```python
from build123d import *

# Parameters (mm, degrees)
F0_R     = 101.6
F1_DEPTH = 25.4


with BuildPart() as f1:
    # F0 (on Front) → F1 (new body)
    with BuildSketch(Plane.XZ):
        Circle(F0_R)
        Polygon((-12.69949, -19.163814), (-12.69949, -0.113814), (-12.69949, 18.936186), (12.70051, 18.936186), (12.7, -19.163814), align=None, mode=Mode.SUBTRACT)
    extrude(amount=F1_DEPTH)


solid = f1.part
```
Check sheet for the modelled part. Datum: model origin and axes. Units: mm. A direction names the side the tool comes from. Coordinates: 2 decimals unless noted, no trailing zeros. Write each loop counter-clockwise with the first axis right and the second up, starting at its lowest first coordinate (ties: lowest second). Pieces come first, ordered by that corner, then holes. Notation, with made-up numbers: (-37.5, -5.5) - (-9.5, -5.5) arc R16 ccw to (-9.5, 12.5) - close; hole circle Ø4 at (7.5, 12.25). An arc over 180 degrees is marked (long way). One line per question, with ' | ' between items.
Item 1: Access from +Z, -Z, +X, -X, +Y, -Y to the whole of each face (thin tool, end or side, straight path). Record for faces 1 (the face through (0, -13, -19.164)), 2 (the face through (21, 0, 1)).
Determined:
face 1: +Y, -Y | face 2: +Z, -Z, +X, -X, +Y
Item 2: Sectioned sample at D-D on z = -77. Record the boundary of the cut face in (x, y), plus the area to 3 significant figures.
Determined:
outline: (-66.28, -25.4) - (66.28, -25.4) - (66.28, 0) - (-66.28, 0) - close | area: 3,370 mm2
Item 3: Gauge pin test, flat ends, axial feed: P1, Ø6, axis at x = -4, z = -16, coming from the +Y side; P2, Ø6, axis at x = -25, z = 21.5, coming from the +Y side; P3, Ø5, axis at y = -10, z = 38.5, coming from the -X side; P4, Ø1.5, axis at x = 36.5, y = -3, coming from the -Z side. Record the tip position at first contact, or that the pin passes through.
Determined:
P1: passes through | P2: stops at y = 0 | P3: stops at x = -95.01 | P4: stops at z = -95.1
Item 4: Sectioned sample at A-A on x = 0. Record the boundary of the cut face in (y, z), plus the area to 3 significant figures.
Determined:
outline: (-25.4, -101.6) - (0, -101.6) - (0, -19.16) - (-25.4, -19.16) - close; (-25.4, 18.94) - (0, 18.94) - (0, 101.6) - (-25.4, 101.6) - close | area: 4,190 mm2
Item 5: Sectioned sample at B-B on z = 0. Record the boundary of the cut face in (x, y), plus the area to 3 significant figures.
Determined:
outline: (-101.6, -25.4) - (-12.7, -25.4) - (-12.7, 0) - (-101.6, 0) - close; (12.7, -25.4) - (101.6, -25.4) - (101.6, 0) - (12.7, 0) - close | area: 4,520 mm2
Item 6: Thickness scan on line 1 (Z direction, x = -18, y = -11.75); line 2 (Z direction, x = -38, y = -11.25); line 3 (X direction, y = -23.25, z = -33). Record the ranges inside material, lowest first. Write a range as [from, to].
Determined:
line 1: z = [-99.99, 99.99] | line 2: z = [-94.23, 94.23] | line 3: x = [-96.09, 96.09]
Item 7: Mould release check, pull along Z, two halves, no side actions. Record for faces 3 (the face through (21, -25.4, 1)), 4 (the face through (-22.025, -12.522, -99.184)), 5 (the face through (0, -13, 18.936)): pulls with the +Z half, pulls with the -Z half, needs draft (parallel to the pull), parting line crosses it, or undercut.
Determined:
face 3: needs draft | face 4: parting line crosses it | face 5: undercut
Item 8: Sectioned sample at C-C on y = -11.5. Record the boundary of the cut face in (x, z).
Determined:
outline: circle Ø203.2 at (0, 0); hole (-12.7, -19.16) - (12.7, -19.16) - (12.7, 18.94) - (-12.7, 18.94) - close
